Input: part model. Units: mm. Frame: model coordinates. A direction names the side the tool comes from. Round coordinates to 2 decimals unless told otherwise and drop trailing zeros. Loops run counter-clockwise (first coordinate to the right, second up) from the corner with the lowest first, then second, coordinate; pieces in that order, holes last. Notation, with made-up numbers: (12.5, 40.5) -> (55.5, 40.5) arc R30 cw to (55.5, 77.5) -> close; hole circle Ø9 at (-34.5, 60). An arc over 180 degrees is marked (long way). One line per question, with ' | ' between items. Start each with the question number.
Q1. Cut plane A-A on y = -15. Return loops of the section in (x, z), and give its area (3 significant figures).
Q2. Cut plane B-B on x = 17.5. Return loops of the section in (y, z), and give its area (4 significant figures).
Q3. Material intervals for L1, parallel to X at y = -14.5, z = 62; L2, parallel to Z at x = 26, y = -23.75; L3, parallel to Y at x = 10, z = 51.5, sorted ascending.
Q4. Access query for faces 1 (the face through (18, -15, 0)), 2 (the face through (27, -8, 50.267)). Directions: +Z, -Z, +X, -X, +Y, -Y. A direction counts if a zero-diameter tool reaches every point of the face in a straight line with its end or side. Return the directions, or none.
Q5. Contact query for flat-ended pins moving along their axis: P1, Ø4, axis at x = 21.5, z = 54.5, coming from the -Y side; P2, Ø6, axis at x = 4, z = 67, coming from the +Y side; P3, Ø6, axis at y = -10, z = 53.5, coming from the -X side. Output: stop coordinate, or through.
Q6. Cut plane C-C on z = 61.5. Return loops of the section in (x, y), and give its area (3 significant figures).
from build123d import *

# Parameters (mm, degrees)
F1_DEPTH = 30
F2_R     = 10.563438
F3_DEPTH = 25


with BuildPart() as f1:
    # F0 (on Front) → F1 (new body)
    with BuildSketch(Plane.XZ):
        Polygon((0, 50.266817), (0, 0), (6.763435, 0), (36.40743, 0), (36.40743, 50.266817), align=None)
    extrude(amount=F1_DEPTH)

    # F2 (on face) → F3 (join)
    with BuildSketch(Plane.XY.offset(50.266817)):
        with Locations((18.203715, -15)):
            Circle(F2_R)
    extrude(amount=F3_DEPTH)


solid = f1.part
Results:
1) outline: (0, 0) -> (36.41, 0) -> (36.41, 50.27) -> (28.77, 50.27) -> (28.77, 75.27) -> (7.64, 75.27) -> (7.64, 50.27) -> (0, 50.27) -> close | area: 2,360 mm^2
2) outline: (-30, 0) -> (0, 0) -> (0, 50.27) -> (-4.46, 50.27) -> (-4.46, 75.27) -> (-25.54, 75.27) -> (-25.54, 50.27) -> (-30, 50.27) -> close | area: 2,035 mm^2
3) L1: 7.65 to 28.76 | L2: 0 to 50.27 | L3: -21.65 to -8.35
4) face 1: -Z, +X, -X, +Y, -Y | face 2: +Z
5) P1: y = -25.48 | P2: through | P3: x = 7.83
6) outline: circle Ø21.13 at (18.2, -15) | area: 351 mm^2
